from build123d import *

# Parameters (mm, degrees)
BOSS_EXTRUDE1_DEPTH = 57
CUT_EXTRUDE1_DEPTH  = 3


with BuildPart() as part:
    # Sketch1 → Boss-Extrude1 (new body)
    with BuildSketch(Plane.XY):
        with BuildLine():
            ThreePointArc((-27.654113618, 27.5), (-39, 0), (-27.654113618, -27.5))
            ThreePointArc((-27.654113618, -27.5), (0, -16), (27.654113618, -27.5))
            ThreePointArc((27.654113618, -27.5), (39, 0), (27.654113618, 27.5))
            ThreePointArc((27.654113618, 27.5), (0, 16), (-27.654113618, 27.5))
        make_face()
    extrude(amount=BOSS_EXTRUDE1_DEPTH)

    # Sketch2 → Cut-Extrude1 (cut)
    with BuildSketch(Plane(origin=(0, 0, 0), x_dir=(-1, 0, 0), z_dir=(0, 0, -1))):
        with BuildLine():
            Line((16, 2), (1.524617098, 5.803063217))
            ThreePointArc((1.524617098, 5.803063217), (0, 6), (-1.524617098, 5.803063217))
            Line((-1.524617098, 5.803063217), (-16, 2))
            ThreePointArc((-16, 2), (-18, 0), (-16, -2))
            Line((-16, -2), (-1.524617098, -5.803063217))
            ThreePointArc((-1.524617098, -5.803063217), (0, -6), (1.524617098, -5.803063217))
            Line((1.524617098, -5.803063217), (16, -2))
            ThreePointArc((16, -2), (18, 0), (16, 2))
        make_face()
    extrude(amount=-CUT_EXTRUDE1_DEPTH, mode=Mode.SUBTRACT)


solid = part.part
Verification items for the finished model (mm, model axes). A direction names the side the tool comes from. Round coordinates to 2 decimals unless told otherwise and drop trailing zeros. Order: outer loops, then holes, each group sorted by start corner. A loop starts at its lowest first (then second) coordinate and runs counter-clockwise, first axis right, second up. Notation, with made-up numbers: (-30, -33.75) -> (5, -33.75) arc R26 ccw to (5, -7.75) -> close; hole circle Ø10 at (-34.75, -33.5). An arc over 180 degrees is marked (long way). Put each result on its own line as item: value.
1) Section check B-B (x = -11). Record the cut outline in (y, z).
Final values:
outline: (-17.58, 0) -> (-3.31, 0) -> (-3.31, 3) -> (3.31, 3) -> (3.31, 0) -> (17.58, 0) -> (17.58, 57) -> (-17.58, 57) -> close
2) Section check A-A (y = 22). Record the cut outline in (x, z).
Final values:
outline: (-32.2, 0) -> (-20.78, 0) -> (-20.78, 57) -> (-32.2, 57) -> close; (20.78, 0) -> (32.2, 0) -> (32.2, 57) -> (20.78, 57) -> close
3) Section check D-D (y = 10). Record the cut outline in (x, z), then the cut area to 3 significant figures.
Final values:
outline: (-37.7, 0) -> (37.7, 0) -> (37.7, 57) -> (-37.7, 57) -> close
area: 4,300 mm^2
4) Set-up check for faces 4 (the cylindrical face through (39, 0, 28)), 5 (the cylindrical face through (18, 0, 1)): record each of +Z, -Z, +X, -X, +Y, -Y from which the full face is reachable in a straight line by a thin tool's end or side.
Final values:
face 4: +Z, -Z, +X
face 5: -Z
5) Mould release check, pull along Y, two halves, no side actions. Record for faces 1 (the cylindrical face through (0, -6, 1)), 2 (the flat face through (-1, 0, 57)), 3 (the cylindrical face through (-39, 0, 28)): +Y half, -Y half, draft (parallel to the pull), parting line (faces both ways), or undercut.
Final values:
face 1: undercut
face 2: draft
face 3: parting line
6) Section check C-C (z = 7). Record the cut outline in (x, y).
Final values:
outline: (-27.65, -27.5) arc R39 cw to (27.65, -27.5) arc R39 ccw to (27.65, 27.5) arc R39 cw to (-27.65, 27.5) arc R39 ccw to start
7) Depth check by flat-ended pin: pin 1 (2 mm diameter, centred on y = 12, z = 9, fed in from -X); pin 2 (5 mm diameter, centred on y = 1.5, z = 28.5, fed in from +X); pin 3 (3 mm diameter, centred on x = 3.5, z = 25.5, fed in from +Y). Enter the tip coordinate at first touch or a pass-through.
Final values:
pin 1: stops at x = -37.42
pin 2: stops at x = 39
pin 3: stops at y = 16.32
8) Material ranges on line 1 (X direction, y = 1, z = 4); line 2 (X direction, y = -23, z = 16.5); line 3 (X direction, y = -19, z = 37.5), recorded low to high.
Final values:
line 1: x = -38.99 to 38.99
line 2: x = -31.5 to -22.29, 22.29 to 31.5
line 3: x = -34.06 to -15, 15 to 34.06
